Input: part model. Units: mm. Frame: model coordinates. Face numbers are marked on the shaded views. A direction names the side the tool comes from. Give positions to 0.01 mm unless a question says otherwise; leave off trailing zeros. Loops run counter-clockwise (first coordinate to the right, second up) from the corner with the lowest first, then second, coordinate; pieces in that order, holes last. Notation, with made-up numbers: M -5,-2.75 L 51,-2.75 A24 cw 51,26.25 Z; hole C 68.25,33 d9. An arc over 180 degrees is marked long. Answer as a JSON object with one key per item and string values. Group by question number.
1) Section query D-D on z = 3.4. Count the separate pieces of the cut face and the enclosed holes in it, plus the area to 3 significant figures.
2) Ray query, L1, parallel to X at y = 17.5, z = 3.75; L2, parallel to Y at x = 7, z = 4.7; L3, parallel to Y at x = -44.5, z = 0.75. Return the intervals inside material, ascending.
3) Section query A-A on y = 15. Return loops of the section in (x, z).
4) Section query C-C on x = -27.5. Return loops of the section in (y, z), plus the area to 3 significant figures.
5) Draft query along X for the marked faces 5, 6, 7 and 8. Return one class per face: +X half, -X half, draft (parallel to the pull), parting line (faces both ways), or undercut.
6) First-contact query: P1, Ø1.8, axis at x = 5.5, z = 3, coming from the -Y side; P2, Ø4, axis at x = 15.01, y = -21.12, coming from the +Z side; P3, Ø1.2, axis at x = -51.93, y = 12.12, coming from the -Z side; P4, Ø1.6, axis at y = -11.5, z = 2, coming from the -X side. Flat tips, straight axial feed; report the tip coordinate or a pass-through.
7) Section query B-B on x = 3. Return loops of the section in (y, z).
8) Access query for the marked faces 1, 2, 3 and 4. Directions: +Z, -Z, +X, -X, +Y, -Y. A direction counts if a zero-diameter tool reaches every point of the face in a straight line with its end or side. Return the directions, or none.
Autodesk Inventor part; units mm, degrees
ref_plane "YZ Plane" through (0, 0, 0) normal (1, 0, 0) x (0, 1, 0)
ref_plane "XZ Plane" through (0, 0, 0) normal (0, 1, 0) x (-1, 0, 0)
ref_plane "XY Plane" through (0, 0, 0) normal (0, 0, 1) x (1, 0, 0)
sketch "Sketch1" plane through (0, 0, 0) normal (0, 0, 1) x (1, 0, 0)
  line L0 (-34.1796, -8.5097) -> (-34.1796, 5.4903)
  line L1 (-34.1796, 5.4903) -> (-17.1796, 5.4903)
  line L2 (-17.1796, 5.4903) -> (-17.1796, -8.5097)
  line L3 (-14.6796, -8.5097) -> (-17.1796, -8.5097)
  line L4 (-14.6796, -13.0097) -> (-14.6796, -8.5097)
  line L5 (-3.6796, -13.0097) -> (-14.6796, -13.0097)
  line L6 (-3.6796, -11.0097) -> (-3.6796, -13.0097)
  arc A0 (-0.6796, -8.0097) -> (-3.6796, -11.0097) centre (-0.6796, -11.0097) ccw
  line L7 (8.3204, -8.0097) -> (-0.6796, -8.0097)
  arc A1 (11.3204, -11.0097) -> (8.3204, -8.0097) centre (8.3204, -11.0097) ccw
  line L8 (11.3204, -20.4968) -> (11.3204, -11.0097)
  arc A2 (11.3204, -20.4968) -> (14.3204, -23.4968) centre (14.3204, -20.4968) ccw
  line L9 (16.3204, -23.4968) -> (14.3204, -23.4968)
  arc A3 (16.3204, -23.4968) -> (19.3204, -20.4968) centre (16.3204, -20.4968) ccw
  line L10 (19.3204, -11.0097) -> (19.3204, -20.4968)
  arc A4 (22.3204, -8.0097) -> (19.3204, -11.0097) centre (22.3204, -11.0097) ccw
  line L11 (26.3204, -8.0097) -> (22.3204, -8.0097)
  arc A5 (26.3204, -8.0097) -> (29.3204, -5.0097) centre (26.3204, -5.0097) ccw
  line L12 (29.3204, 24.9903) -> (29.3204, -5.0097)
  arc A6 (29.3204, 24.9903) -> (23.3204, 30.9903) centre (23.3204, 24.9903) ccw
  line L13 (-2.1796, 30.9903) -> (23.3204, 30.9903)
  line L14 (-2.1796, 28.9903) -> (-2.1796, 30.9903)
  line L15 (-49.1796, 28.9903) -> (-2.1796, 28.9903)
  line L16 (-49.1796, 30.9903) -> (-49.1796, 28.9903)
  arc A7 (-49.1796, 30.9903) -> (-54.6796, 25.0112) centre (-48.6796, 25.0112) ccw
  line L17 (-54.6796, -5.0097) -> (-54.6796, 25.0112)
  arc A8 (-54.6796, -5.0097) -> (-51.6796, -8.0097) centre (-51.6796, -5.0097) ccw
  line L18 (-50.6796, -8.0097) -> (-51.6796, -8.0097)
  arc A9 (-47.6796, -11.0097) -> (-50.6796, -8.0097) centre (-50.6796, -11.0097) ccw
  line L19 (-47.6796, -13.0097) -> (-47.6796, -11.0097)
  line L20 (-36.6796, -13.0097) -> (-47.6796, -13.0097)
  line L21 (-36.6796, -8.5097) -> (-36.6796, -13.0097)
  line L22 (-34.1796, -8.5097) -> (-36.6796, -8.5097)
  circle A10 centre (15.0119, -15.1214) radius 1.5
  circle A11 centre (15.0119, -21.1214) radius 1.5
  circle A12 centre (-51.9296, 20.6159) radius 0.75
  circle A13 centre (-51.9296, 12.1159) radius 0.75
  circle A14 centre (-45.6796, 8.2799) radius 0.75
  circle A15 centre (-48.6796, 26.9903) radius 1.5
  circle A16 centre (26.3204, -5.0097) radius 1.5
  circle A17 centre (-14.1796, -2.0097) radius 1.5
  circle A18 centre (-51.6796, -5.0097) radius 1.5
  circle A19 centre (20.3204, 26.4903) radius 1.5
  circle A20 centre (-37.1796, -2.0097) radius 1.5
  line L23 (-49.6796, 10.1903) -> (-49.6796, 20.7903)
  line L24 (-49.6796, 20.7903) -> (-25.6796, 20.7903)
  line L25 (-25.6796, 20.7903) -> (-25.6796, 10.1903)
  line L26 (-25.6796, 10.1903) -> (-49.6796, 10.1903)
  line L27 (0.3204, 20.7903) -> (24.3204, 20.7903)
  line L28 (24.3204, 20.7903) -> (24.3204, 10.1903)
  line L29 (24.3204, 10.1903) -> (0.3204, 10.1903)
  line L30 (0.3204, 10.1903) -> (0.3204, 20.7903)
  point P0 (0, 0)
  point P1 (0, 0)
extrude "Extrusion1" add sketch "Sketch1" along normal blind 6
properties part number "XcrRight_a"
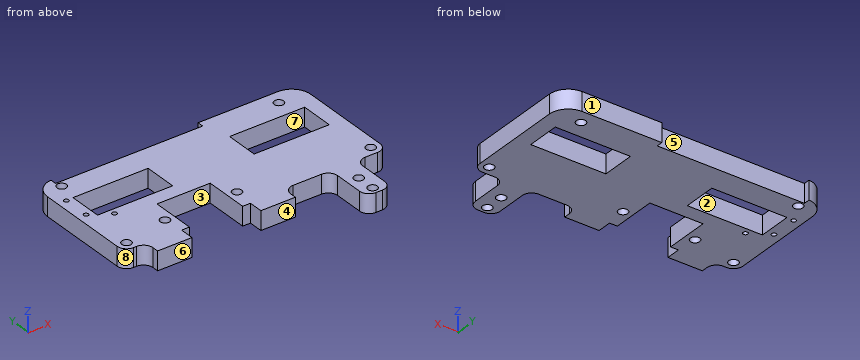
Output:
{
 "1": {"separate pieces": "1", "enclosed holes": "13", "area": "2,600 mm^2"},
 "2": {"L1": "x = -54.68 to -49.68, -25.68 to 0.32, 24.32 to 29.32", "L2": "y = -8.01 to 10.19, 20.79 to 30.99", "L3": "y = -13.01 to 10.19, 20.79 to 28.99"},
 "3": {"outline": "M -54.68,0 L -49.68,0 L -49.68,6 L -54.68,6 Z; M -25.68,0 L 0.32,0 L 0.32,6 L -25.68,6 Z; M 24.32,0 L 29.32,0 L 29.32,6 L 24.32,6 Z"},
 "4": {"outline": "M 5.49,0 L 10.19,0 L 10.19,6 L 5.49,6 Z; M 20.79,0 L 28.99,0 L 28.99,6 L 20.79,6 Z", "area": "77.4 mm^2"},
 "5": {"face 5": "undercut", "face 6": "draft", "face 7": "undercut", "face 8": "-X half"},
 "6": {"P1": "stops at y = -8.01", "P2": "stops at z = 6", "P3": "passes through", "P4": "stops at x = -47.7"},
 "7": {"outline": "M -8.01,0 L 10.19,0 L 10.19,6 L -8.01,6 Z; M 20.79,0 L 30.99,0 L 30.99,6 L 20.79,6 Z"},
 "8": {"face 1": "+Z, -Z, +X, -X, +Y", "face 2": "+Z, -Z", "face 3": "+Z, -Z, -Y", "face 4": "+Z, -Z, -X, -Y"}
}
